from build123d import *

# Parameters (mm, degrees)
BOSS_EXTRUDE1_START  = -0.825
BOSS_EXTRUDE1_DEPTH  = 1.65
BOSS_EXTRUDE2_START  = 1.105
BOSS_EXTRUDE2_DEPTH  = 1.105
BOSS_EXTRUDE3_DEPTH  = 1.105
CUT_EXTRUDE1_DEPTH   = 1.65
SKETCH5_W            = 9.85
SKETCH5_H            = 7.65
BOSS_EXTRUDE4_DEPTH  = 7.55
CUT_EXTRUDE2_REACH   = 15.28
SKETCH6_W            = 1.65
SKETCH6_H            = 5.3
SKETCH7_W            = 3.86
SKETCH7_H            = 2.52
BOSS_EXTRUDE5_DEPTH  = 4
SKETCH8_W            = 1.65
SKETCH8_H            = 9.3
CUT_EXTRUDE3_DEPTH   = 0.9
SKETCH9_W            = 0.7
SKETCH9_H            = 6.63
CUT_EXTRUDE4_DEPTH   = 15.996819663
BOSS_EXTRUDE6_DEPTH  = 6.63
CUT_EXTRUDE5_DEPTH   = 14.226552839
SKETCH12_W           = 2.4
SKETCH12_H           = 2.4
BOSS_EXTRUDE7_DEPTH  = 6.35
SKETCH13_W           = 1.47
SKETCH13_H           = 1.5
CUT_EXTRUDE6_DEPTH   = 1
SKETCH14_W           = 2.4
SKETCH14_H           = 2.4
BOSS_EXTRUDE8_DEPTH  = 6.35
SKETCH15_W           = 1.47
SKETCH15_H           = 1.5
CUT_EXTRUDE7_DEPTH   = 1
SKETCH16_W           = 2.4
SKETCH16_H           = 2.4
BOSS_EXTRUDE9_DEPTH  = 6.35
SKETCH17_W           = 1.47
SKETCH17_H           = 1.5
CUT_EXTRUDE8_DEPTH   = 1
SKETCH18_W           = 2.4
SKETCH18_H           = 2.4
BOSS_EXTRUDE10_DEPTH = 6.35
SKETCH19_W           = 1.47
SKETCH19_H           = 1.5
CUT_EXTRUDE9_DEPTH   = 1
SKETCH20_W           = 2.4
SKETCH20_H           = 2.4
BOSS_EXTRUDE11_DEPTH = 6.35
SKETCH21_W           = 1.47
SKETCH21_H           = 1.5
CUT_EXTRUDE10_DEPTH  = 1
SKETCH22_W           = 2.4
SKETCH22_H           = 2.4
BOSS_EXTRUDE12_DEPTH = 6.35
SKETCH23_W           = 1.47
SKETCH23_H           = 1.5
CUT_EXTRUDE11_DEPTH  = 1
SKETCH24_W           = 2.49
SKETCH24_H           = 2.49
CUT_EXTRUDE12_DEPTH  = 1
SKETCH25_W           = 2.49
SKETCH25_H           = 2.49
CUT_EXTRUDE13_DEPTH  = 1
SKETCH26_W           = 2.49
SKETCH26_H           = 2.49
CUT_EXTRUDE14_DEPTH  = 1
SKETCH27_W           = 2.49
SKETCH27_H           = 2.49
CUT_EXTRUDE15_DEPTH  = 1
SKETCH28_W           = 2.49
SKETCH28_H           = 2.49
CUT_EXTRUDE16_DEPTH  = 1
SKETCH29_W           = 2.29
SKETCH29_H           = 1.02
BOSS_EXTRUDE13_DEPTH = 0.7
SKETCH30_W           = 2.3
SKETCH30_H           = 1.02
BOSS_EXTRUDE14_DEPTH = 0.7
SKETCH31_W           = 2.49
SKETCH31_H           = 2.49
CUT_EXTRUDE17_DEPTH  = 1
CHAMFER1_SIZE        = 0.6
CHAMFER2_SIZE        = 0.25
FILLET1_R            = 0.25
FILLET2_R            = 0.15


with BuildPart() as part:
    # Boss-Extrude1: read off the stored shape, not the designer's step
    # Boss-Extrude1 outline → Boss-Extrude1 (new body)
    with BuildSketch(Plane.YZ.offset(BOSS_EXTRUDE1_START)):
        with BuildLine():
            Line((2.98, -3.42), (1.55, -3.42))
            Line((1.55, -3.42), (1.55, -6.7))
            Line((1.55, -6.7), (9.11, -6.7))
            Line((9.11, -6.7), (9.11, -4.98))
            Line((9.11, -4.98), (8.11, -3.98))
            Line((8.11, -3.98), (2.98, -3.98))
            ThreePointArc((2.98, -3.98), (2.7, -3.7), (2.98, -3.42))
        make_face()
    extrude(amount=BOSS_EXTRUDE1_DEPTH)

    # Sketch2 → Boss-Extrude2 (add)
    with BuildSketch(Plane.ZY.offset(0.825).offset(BOSS_EXTRUDE2_START)):
        with BuildLine():
            Line((-6.7, 1.55), (-6.7, 9.11))
            Line((-6.7, 9.11), (-4.98, 9.11))
            Line((-4.98, 9.11), (-3.98, 8.11))
            Line((-3.98, 8.11), (-3.98, 2.98))
            ThreePointArc((-3.98, 2.98), (-3.7, 2.7), (-3.42, 2.98))
            Line((-3.42, 2.98), (-3.42, 1.55))
            Line((-3.42, 1.55), (-6.7, 1.55))
        make_face()
    extrude(amount=-BOSS_EXTRUDE2_DEPTH)

    # Sketch3 → Boss-Extrude3 (add)
    with BuildSketch(Plane(origin=(0.825, 0, 0), x_dir=(0, 0, -1), z_dir=(1, 0, 0))):
        with BuildLine():
            Line((6.7, 1.55), (3.42, 1.55))
            Line((3.42, 1.55), (3.42, 2.98))
            ThreePointArc((3.42, 2.98), (3.7, 2.7), (3.98, 2.98))
            Line((3.98, 2.98), (3.98, 8.11))
            Line((3.98, 8.11), (4.98, 9.11))
            Line((4.98, 9.11), (6.7, 9.11))
            Line((6.7, 9.11), (6.7, 1.55))
        make_face()
    extrude(amount=BOSS_EXTRUDE3_DEPTH)

    # Sketch4 → Cut-Extrude1 (cut)
    with BuildSketch(Plane(origin=(-0.825, 0, 0), x_dir=(0, -1, 0), z_dir=(-1, 0, 0))):
        with BuildLine():
            Line((-2.98, -3.98), (-1.55, -3.98))
            Line((-1.55, -3.98), (-1.55, -3.42))
            Line((-1.55, -3.42), (-2.98, -3.42))
            ThreePointArc((-2.98, -3.42), (-2.7, -3.7), (-2.98, -3.98))
        make_face()
    extrude(amount=-CUT_EXTRUDE1_DEPTH, mode=Mode.SUBTRACT)

    # Sketch5 → Boss-Extrude4 (add)
    with BuildSketch(Plane(origin=(0, 0, -3.42), x_dir=(-1, 0, 0), z_dir=(0, 0, -1))):
        with Locations((0.005, -0.175)):
            Rectangle(SKETCH5_W, SKETCH5_H)
    extrude(amount=-BOSS_EXTRUDE4_DEPTH)

    # Sketch6 → Cut-Extrude2 (cut, up to next)
    with BuildSketch(Plane(origin=(0, 0, -4.18), x_dir=(-1, 0, 0), z_dir=(0, 0, -1)), mode=Mode.PRIVATE) as cut_extrude2_sk1:
        with Locations((0, 4.2)):
            Rectangle(SKETCH6_W, SKETCH6_H)
    cut_extrude2_tool1 = extrude(cut_extrude2_sk1.sketch, amount=-CUT_EXTRUDE2_REACH, mode=Mode.PRIVATE) & part.part
    add(cut_extrude2_tool1.solids().sort_by_distance((0, 4.2, -4.18))[0], mode=Mode.SUBTRACT)

    # Sketch7 → Boss-Extrude5 (add)
    with BuildSketch(Plane.XZ.offset(-1.55)):
        with Locations((0, -5.44)):
            Rectangle(SKETCH7_W, SKETCH7_H)
    extrude(amount=BOSS_EXTRUDE5_DEPTH)

    # Sketch8 → Cut-Extrude3 (cut)
    with BuildSketch(Plane.XY.offset(-4.18)):
        with Locations((0, 2.2)):
            Rectangle(SKETCH8_W, SKETCH8_H)
    extrude(amount=-CUT_EXTRUDE3_DEPTH, mode=Mode.SUBTRACT)

    # Sketch9 → Cut-Extrude4 (cut, through all)
    with BuildSketch(Plane.ZY.offset(4.93)):
        with Locations((3.78, 0.335)):
            Rectangle(SKETCH9_W, SKETCH9_H)
    extrude(amount=-CUT_EXTRUDE4_DEPTH, mode=Mode.SUBTRACT)

    # Sketch10 → Boss-Extrude6 (add)
    with BuildSketch(Plane(origin=(0, -2.98, 0), x_dir=(-1, 0, 0), z_dir=(0, 1, 0))):
        with BuildLine():
            Line((3.34, 3.43), (2.74, 3.43))
            ThreePointArc((2.74, 3.43), (3.04, 3.73), (3.34, 3.43))
        make_face()
    extrude(amount=BOSS_EXTRUDE6_DEPTH)

    # Sketch11 → Cut-Extrude5 (cut, through all)
    with BuildSketch(Plane(origin=(1.93, 0, 0), x_dir=(0, 0, -1), z_dir=(1, 0, 0))):
        Polygon((5.68, -0.43), (6.7, -1.45), (6.7, 9.11), (5.68, 9.11), align=None)
    extrude(amount=-CUT_EXTRUDE5_DEPTH, mode=Mode.SUBTRACT)

    # Sketch12 → Boss-Extrude7 (add)
    with BuildSketch(Plane(origin=(0, 3.65, 0), x_dir=(-1, 0, 0), z_dir=(0, 1, 0))):
        with Locations((3, 1.5)):
            Rectangle(SKETCH12_W, SKETCH12_H)
    extrude(amount=BOSS_EXTRUDE7_DEPTH)

    # Sketch13 → Cut-Extrude6 (cut)
    with BuildSketch(Plane(origin=(0, 10, 0), x_dir=(-1, 0, 0), z_dir=(0, 1, 0))):
        with Locations((3, 1.51)):
            Rectangle(SKETCH13_W, SKETCH13_H)
    extrude(amount=-CUT_EXTRUDE6_DEPTH, mode=Mode.SUBTRACT)

    # Sketch14 → Boss-Extrude8 (add)
    with BuildSketch(Plane(origin=(0, 3.65, 0), x_dir=(-1, 0, 0), z_dir=(0, 1, 0))):
        with Locations((0, 1.5)):
            Rectangle(SKETCH14_W, SKETCH14_H)
    extrude(amount=BOSS_EXTRUDE8_DEPTH)

    # Sketch15 → Cut-Extrude7 (cut)
    with BuildSketch(Plane(origin=(0, 10, 0), x_dir=(-1, 0, 0), z_dir=(0, 1, 0))):
        with Locations((0, 1.51)):
            Rectangle(SKETCH15_W, SKETCH15_H)
    extrude(amount=-CUT_EXTRUDE7_DEPTH, mode=Mode.SUBTRACT)

    # Sketch16 → Boss-Extrude9 (add)
    with BuildSketch(Plane(origin=(0, 3.65, 0), x_dir=(-1, 0, 0), z_dir=(0, 1, 0))):
        with Locations((0, -1.5)):
            Rectangle(SKETCH16_W, SKETCH16_H)
    extrude(amount=BOSS_EXTRUDE9_DEPTH)

    # Sketch17 → Cut-Extrude8 (cut)
    with BuildSketch(Plane(origin=(0, 10, 0), x_dir=(-1, 0, 0), z_dir=(0, 1, 0))):
        with Locations((0, -1.49)):
            Rectangle(SKETCH17_W, SKETCH17_H)
    extrude(amount=-CUT_EXTRUDE8_DEPTH, mode=Mode.SUBTRACT)

    # Sketch18 → Boss-Extrude10 (add)
    with BuildSketch(Plane(origin=(0, 3.65, 0), x_dir=(-1, 0, 0), z_dir=(0, 1, 0))):
        with Locations((-3, 1.5)):
            Rectangle(SKETCH18_W, SKETCH18_H)
    extrude(amount=BOSS_EXTRUDE10_DEPTH)

    # Sketch19 → Cut-Extrude9 (cut)
    with BuildSketch(Plane(origin=(0, 10, 0), x_dir=(-1, 0, 0), z_dir=(0, 1, 0))):
        with Locations((-3, 1.51)):
            Rectangle(SKETCH19_W, SKETCH19_H)
    extrude(amount=-CUT_EXTRUDE9_DEPTH, mode=Mode.SUBTRACT)

    # Sketch20 → Boss-Extrude11 (add)
    with BuildSketch(Plane(origin=(0, 3.65, 0), x_dir=(-1, 0, 0), z_dir=(0, 1, 0))):
        with Locations((-3, -1.5)):
            Rectangle(SKETCH20_W, SKETCH20_H)
    extrude(amount=BOSS_EXTRUDE11_DEPTH)

    # Sketch21 → Cut-Extrude10 (cut)
    with BuildSketch(Plane(origin=(0, 10, 0), x_dir=(-1, 0, 0), z_dir=(0, 1, 0))):
        with Locations((-3, -1.49)):
            Rectangle(SKETCH21_W, SKETCH21_H)
    extrude(amount=-CUT_EXTRUDE10_DEPTH, mode=Mode.SUBTRACT)

    # Sketch22 → Boss-Extrude12 (add)
    with BuildSketch(Plane(origin=(0, 3.65, 0), x_dir=(-1, 0, 0), z_dir=(0, 1, 0))):
        with Locations((3, -1.5)):
            Rectangle(SKETCH22_W, SKETCH22_H)
    extrude(amount=BOSS_EXTRUDE12_DEPTH)

    # Sketch23 → Cut-Extrude11 (cut)
    with BuildSketch(Plane(origin=(0, 10, 0), x_dir=(-1, 0, 0), z_dir=(0, 1, 0))):
        with Locations((3, -1.49)):
            Rectangle(SKETCH23_W, SKETCH23_H)
    extrude(amount=-CUT_EXTRUDE11_DEPTH, mode=Mode.SUBTRACT)

    # Sketch24 → Cut-Extrude12 (cut)
    with BuildSketch(Plane.XZ.offset(4)):
        with Locations((-3, -1.375)):
            Rectangle(SKETCH24_W, SKETCH24_H)
    extrude(amount=-CUT_EXTRUDE12_DEPTH, mode=Mode.SUBTRACT)

    # Sketch25 → Cut-Extrude13 (cut)
    with BuildSketch(Plane.XZ.offset(4)):
        with Locations((-3, 1.625)):
            Rectangle(SKETCH25_W, SKETCH25_H)
    extrude(amount=-CUT_EXTRUDE13_DEPTH, mode=Mode.SUBTRACT)

    # Sketch26 → Cut-Extrude14 (cut)
    with BuildSketch(Plane.XZ.offset(4)):
        with Locations((0, -1.375)):
            Rectangle(SKETCH26_W, SKETCH26_H)
    extrude(amount=-CUT_EXTRUDE14_DEPTH, mode=Mode.SUBTRACT)

    # Sketch27 → Cut-Extrude15 (cut)
    with BuildSketch(Plane.XZ.offset(4)):
        with Locations((0, 1.625)):
            Rectangle(SKETCH27_W, SKETCH27_H)
    extrude(amount=-CUT_EXTRUDE15_DEPTH, mode=Mode.SUBTRACT)

    # Sketch28 → Cut-Extrude16 (cut)
    with BuildSketch(Plane.XZ.offset(4)):
        with Locations((3, -1.375)):
            Rectangle(SKETCH28_W, SKETCH28_H)
    extrude(amount=-CUT_EXTRUDE16_DEPTH, mode=Mode.SUBTRACT)

    # Sketch29 → Boss-Extrude13 (add)
    with BuildSketch(Plane(origin=(0, 0, -3.42), x_dir=(-1, 0, 0), z_dir=(0, 0, -1))):
        with Locations((-3.775, -3.49)):
            Rectangle(SKETCH29_W, SKETCH29_H)
    extrude(amount=BOSS_EXTRUDE13_DEPTH)

    # Sketch30 → Boss-Extrude14 (add)
    with BuildSketch(Plane(origin=(0, 0, -3.42), x_dir=(-1, 0, 0), z_dir=(0, 0, -1))):
        with Locations((3.78, -3.49)):
            Rectangle(SKETCH30_W, SKETCH30_H)
    extrude(amount=BOSS_EXTRUDE14_DEPTH)

    # Sketch31 → Cut-Extrude17 (cut)
    with BuildSketch(Plane.XZ.offset(4)):
        with Locations((3, 1.625)):
            Rectangle(SKETCH31_W, SKETCH31_H)
    extrude(amount=-CUT_EXTRUDE17_DEPTH, mode=Mode.SUBTRACT)

    # Chamfer1
    chamfer1_edges = [part.edges().sort_by_distance(p)[0] for p in [
        (-1.8, 6.825, 2.7),
        (1.2, 6.825, 2.7),
        (1.2, 6.825, -0.3),
        (4.2, 6.825, 2.7),
        (4.2, 6.825, -0.3),
        (-4.2, 6.825, -0.3),
    ]]
    chamfer(chamfer1_edges, length=CHAMFER1_SIZE)

    # Chamfer2
    chamfer2_edges = [part.edges().sort_by_distance(p)[0] for p in [
        (-2.265, 9.5, 2.26),
        (-3.735, 9.5, 2.26),
        (0.735, 9.5, 2.26),
        (-0.735, 9.5, 2.26),
        (0.735, 9.5, -0.74),
        (-0.735, 9.5, -0.74),
        (3.735, 9.5, 2.26),
        (2.265, 9.5, 2.26),
        (3.735, 9.5, -0.74),
        (2.265, 9.5, -0.74),
        (-2.265, 9.5, -0.74),
        (-3.735, 9.5, -0.74),
    ]]
    chamfer(chamfer2_edges, length=CHAMFER2_SIZE)

    # Fillet1
    fillet1_edges = [part.edges().sort_by_distance(p)[0] for p in [
        (-1.93, 2.265, -3.42),
        (1.93, 2.265, -3.42),
        (-0.005, -2.98, 4.13),
        (3.775, -2.98, -4.12),
        (-3.78, -2.98, -4.12),
    ]]
    fillet(fillet1_edges, radius=FILLET1_R - 0.0001)  # a hair under: the kernel refuses the full size

    # Fillet2
    fillet2_edges = [part.edges().sort_by_distance(p)[0] for p in [
        (1.3775, 1.55, -4.18),
        (-1.3775, 1.55, -4.18),
    ]]
    fillet(fillet2_edges, radius=FILLET2_R)


solid = part.part
Verification items for the finished model (mm, model axes). A direction names the side the tool comes from. Give positions to 0.01 mm unless a question says otherwise; leave off trailing zeros. Write each loop counter-clockwise with the first axis right and the second up, starting at its lowest first coordinate (ties: lowest second). Pieces come first, ordered by that corner, then holes. Notation, with made-up numbers: (-31.5, 66) -> (3.5, 66) arc R18 cw to (3.5, 74) -> close; hole circle Ø10 at (9.25, -36.75). An arc over 180 degrees is marked (long way). Use CSV: the item, a comma, the result in double quotes.
(1) Sectioned sample at B-B (x = -4). Record the cut outline in (y, z).
Derived:
outline,"(-4, -4.12) -> (-3.23, -4.12) arc R0.25 ccw to (-2.98, -3.87) -> (-2.98, -3.42) -> (3.65, -3.42) -> (3.65, -2.7) -> (10, -2.7) -> (10, -0.7) -> (3.65, -0.7) -> (3.65, 0.3) -> (10, 0.3) -> (10, 2.7) -> (3.65, 2.7) -> (3.65, 3.43) -> (-2.98, 3.43) -> (-2.98, 3.88) arc R0.25 ccw to (-3.23, 4.13) -> (-4, 4.13) -> (-4, 2.87) -> (-3, 2.87) -> (-3, 0.38) -> (-4, 0.38) -> (-4, -0.13) -> (-3, -0.13) -> (-3, -2.62) -> (-4, -2.62) -> close"
(2) Set-up check for faces 1 (the flat face through (-1.2, 7, 1)), 2 (the flat face through (3, -3.5, -0.13)), 3 (the flat face through (-3, 7, 2.7)): record each of +Z, -Z, +X, -X, +Y, -Y from which the full face is reachable in a straight line by a thin tool's end or side.
Derived:
face 1,"+Z, +Y"
face 2,"-Y"
face 3,"+Z, +X, -X, +Y"
(3) Go/stop test with flat-tipped pins: pin 1 (2 mm diameter, centred on x = -1.5, y = 3.5, fed in from +Z); pin 2 (1.5 mm diameter, centred on x = -3.5, y = 3, fed in from +Z); pin 3 (0.8 mm diameter, centred on x = -3.5, y = -3.5, fed in from -Z). Record where each tip stops, or that it passes through.
Derived:
pin 1,"stops at z = 3.43"
pin 2,"stops at z = 3.73"
pin 3,"stops at z = -4.12"
(4) Sectioned sample at D-D (z = -5.25). Record the cut outline in (x, y), plus the area to 3 significant figures.
Derived:
outline,"(-1.93, -2.45) -> (1.93, -2.45) -> (1.93, 9.11) -> (-1.93, 9.11) -> close"
area,"44.6 mm^2"
(5) Sectioned sample at A-A (y = -0.75). Record the cut outline in (x, z) (3 decimals).
Derived:
outline,"(-4.93, -3.42) -> (4.92, -3.42) -> (4.92, 3.43) -> (-2.74, 3.43) arc R0.3 ccw to (-3.34, 3.43) -> (-4.93, 3.43) -> close; (-1.93, -6) -> (1.93, -6) -> (1.93, -4.18) -> (0.825, -4.18) -> (0.825, -5.08) -> (-0.825, -5.08) -> (-0.825, -4.18) -> (-1.93, -4.18) -> close"
(6) Release check for a two-part mould opening along X. For faces 4 (the flat face through (0, -3.5, 2.87)), 5 (the flat face through (4.2, 7, -2)), 6 (the flat face through (3, 7, 2.7)) record: +X half, -X half, draft (parallel to the pull), parting line (faces both ways), or undercut.
Derived:
face 4,"undercut"
face 5,"+X half"
face 6,"draft"
(7) Sectioned sample at C-C (y = 2). Record the cut outline in (x, z) (3 decimals).
Derived:
outline,"(-4.93, -3.42) -> (-2.18, -3.42) arc R0.25 cw to (-1.93, -3.67) -> (-1.93, -5.68) -> (1.93, -5.68) -> (1.93, -3.67) arc R0.25 cw to (2.18, -3.42) -> (4.92, -3.42) -> (4.92, 3.43) -> (-2.74, 3.43) arc R0.3 ccw to (-3.34, 3.43) -> (-4.93, 3.43) -> close; hole (-0.825, -5.08) -> (0.825, -5.08) -> (0.825, -3.42) -> (-0.825, -3.42) -> close"
(8) Material ranges on L1, parallel to X at y = 6.5, z = -1; L2, parallel to Z at x = 0.75, y = -2; L3, parallel to Z at x = -1.75, y = -0.25, recorded low to high.
Derived:
L1,"x = -4.2 to -1.8, -1.2 to 1.2, 1.8 to 4.2"
L2,"z = -6.7 to -5.08, -3.42 to 3.43"
L3,"z = -5.68 to -4.18, -3.42 to 3.43"
